```python
from build123d import *

# Parameters (mm, degrees)
BOSS_EXTRUDE1_DEPTH = 17


with BuildPart() as part:
    # Sketch1 → Revolve1 (revolve)
    with BuildSketch(Plane(origin=(0, 0, 0), x_dir=(0, 0, -1), z_dir=(1, 0, 0)), mode=Mode.PRIVATE) as revolve1_sk:
        Polygon((-22.55, 0), (-22.55, 1.59), (-9.95, 1.59), (-9.95, 10.926977996), (-7.45, 14), (-3.95, 14), (-3.95, 1.59), (-3.45, 1.59), (-3.45, 14), (15.65, 14), (21.05, 6.187841706), (21.05, 4), (21.652703363, 4), (22.55, 2.589018231), (22.55, 1.660098946), (22.479901054, 1.59), (22.55, 1.519901054), (22.55, 0), align=None)
    revolve(revolve1_sk.sketch.rotate(Axis((0, 0, 22.55), (0, 0, -1)), 180), axis=Axis((0, 0, 22.55), (0, 0, -1)))

    # Sketch2 → Boss-Extrude1 (add)
    with BuildSketch(Plane(origin=(0, 0, 0), x_dir=(0, 0, -1), z_dir=(1, 0, 0))):
        with BuildLine():
            Line((-4.658936123, 2.4), (-4.658936123, -2.4))
            ThreePointArc((-4.658936123, -2.4), (-5.908936123, -3.65), (-7.158936123, -2.4))
            Line((-7.158936123, -2.4), (-7.158936123, 2.4))
            ThreePointArc((-7.158936123, 2.4), (-5.908936123, 3.65), (-4.658936123, 2.4))
        make_face()
    extrude(amount=BOSS_EXTRUDE1_DEPTH)


solid = part.part
```
Geometry check sheet. Reference: the model listing, model coordinates, mm. A direction names the side the tool comes from. Coordinates: 2 decimals unless noted, no trailing zeros. Order: outer loops, then holes, each group sorted by start corner. A loop starts at its lowest first (then second) coordinate and runs counter-clockwise, first axis right, second up.
Item 1: Scan lines: line 1 along Z through (x, y) = (2.5, 4.75); line 2 along Z through (x, y) = (1, 1.75); line 3 along X through (y, z) = (3, -16.5). Record each from-to range of solid material in increasing order.
Item 2: Depth check by flat-ended pin: pin 1 (1.6 mm diameter, centred on x = 15, y = 0, fed in from +Z); pin 2 (10 mm diameter, centred on x = -6.5, z = -9.5, fed in from +Y); pin 3 (6 mm diameter, centred on y = 4.5, z = -10.5, fed in from -X). Enter the tip coordinate at first touch or a pass-through.
Item 3: Section check C-C (z = 2). Enter the section's corners in (x, y), plus the area to 3 significant figures.
Item 4: Tool access check on faces 1 (the cylindrical face through (3.905, 0.867, -21.356)), 2 (the cylindrical face through (0.97, 1.26, 16.16)), 3 (the cylindrical face through (15.23, -3.65, 5.88)), 4 (the cylindrical face through (0.97, 1.26, 3.7)), 5 (the flat face through (17, 0, 6)). Record the directions out of +Z, -Z, +X, -X, +Y, -Y that give a thin tool (end or side, any length) a straight path to the whole face; none if there is none.
Item 5: Section check B-B (z = 13). Enter the section's corners in (x, y), plus the area to 3 significant figures.
Check sheet entries:
1. line 1: z = -21.05 to 3.45, 3.95 to 9.95
1. line 2: z = -22.55 to 3.45, 3.95 to 9.95
1. line 3: x = -12.41 to 12.41
2. pin 1: stops at z = 7.16
2. pin 2: stops at y = 13.92
2. pin 3: stops at x = -13.92
3. outline: circle Ø28 at (0, 0)
3. area: 616 mm2
4. face 1: -Z
4. face 2: +Z
4. face 3: +X, -Y
4. face 4: none
4. face 5: +Z, -Z, +X, +Y, -Y
5. outline: circle Ø3.18 at (0, 0)
5. area: 7.94 mm2
